Autodesk Inventor part; units mm, degrees
ref_plane "工作平面2" through (0, 56, 0) normal (0, 1, 0) x (1, 0, 0)
ref_plane "YZ Plane" through (0, 0, 0) normal (1, 0, 0) x (0, 1, 0)
ref_plane "XZ Plane" through (0, 0, 0) normal (0, 1, 0) x (-1, 0, 0)
sketch "草图1" plane through (0, 0, 0) normal (0, 1, 0) x (-1, 0, 0)
  circle A0 centre (0, 0) radius 35.5
  dimension "d0" = 71
extrude "拉伸1" add sketch "草图1" along normal blind 3
sketch "草图2" plane through (0, 3, 0) normal (0, 1, 0) x (1, 0, 0)
  circle A0 centre (0, 0) radius 15.5
  circle A1 centre (0, 0) radius 12.5
  dimension "d3" = 31
  dimension "d4" = 25
extrude "拉伸2" add sketch "草图2" along normal blind 41
sketch "草图3" plane through (0, 44, 0) normal (0, 1, 0) x (1, 0, 0)
  circle A0 centre (0, 0) radius 30
  dimension "d7" = 60
extrude "拉伸3" add sketch "草图3" along normal blind 3
sketch "草图4" plane through (0, 0, 0) normal (0, -1, 0) x (1, 0, 0)
  circle A0 centre (0, 0) radius 12.5
extrude "拉伸4" cut sketch "草图4" against normal blind 3
sketch "草图5" plane through (0, 47, 0) normal (0, 1, 0) x (1, 0, 0)
  circle A0 centre (0, 0) radius 12.5
  circle A1 centre (0, 0) radius 3.5
  dimension "d12" = 7
extrude "拉伸5" cut sketch "草图5" against normal blind 5 contours A1
sketch "草图6" plane through (0, 47, 0) normal (0, 1, 0) x (1, 0, 0)
  circle A0 centre (0, 0) radius 10
  circle A1 centre (0, 0) radius 22.5
  dimension "d15" = 20
  dimension "d16" = 45
extrude "拉伸6" add sketch "草图6" along normal blind 10
sketch "草图7" plane through (0, 47, 0) normal (0, 1, 0) x (1, 0, 0)
  circle A0 centre (0, 0) radius 3.5
  line L0 (3.5, 3.5) -> (48.5, 3.5)
  line L1 (48.5, 3.5) -> (48.5, -3.5)
  line L2 (48.5, -3.5) -> (3.5, -3.5)
  line L3 (3.5, -3.5) -> (3.5, 3.5)
  dimension "d19" = 45
  dimension "d20" = 7
extrude "拉伸7" [suppressed]
sketch "草图8" plane through (0, 47, 0) normal (0, 1, 0) x (1, 0, 0)
  circle A0 centre (44.1819, 0) radius 2.5
  point P0 (0, 0)
  dimension "d23" = 5
extrude "拉伸8" [suppressed]
pattern_circular "环形阵列1" [suppressed]
sketch "草图9" plane through (0, 47, 0) normal (0, 1, 0) x (1, 0, 0)
  line L0 (24, -2.5) -> (29, -2.5)
  line L1 (29, -2.5) -> (29, 2.5)
  line L2 (29, 2.5) -> (24, 2.5)
  line L3 (24, 2.5) -> (24, -2.5)
  line L4 (-49.7, 0) -> (49.7, 0)
  point P0 (0, 0)
  dimension "d32" = 5
  dimension "d33" = 5
  dimension "d34" = 24
extrude "拉伸9" add sketch "草图9" along normal blind 16
sketch "草图10" plane through (0, 44, 0) normal (0, -1, 0) x (1, 0, 0)
  line L0 (13.5, 10) -> (26.5, 10)
  line L1 (26.5, 10) -> (26.5, -12)
  line L2 (26.5, -12) -> (13.5, -12)
  line L3 (13.5, -12) -> (13.5, 10)
  point P0 (0, 0)
  dimension "d36" = 10
  dimension "d38" = 22
  dimension "d40" = 13
  dimension "d41" = 13.5
extrude "拉伸10" cut sketch "草图10" along normal blind 4
sketch "草图11" plane through (0, 44, 0) normal (0, -1, 0) x (1, 0, 0)
  circle A0 centre (0, 0) radius 12.5
  line L0 (24, 2.5) -> (29, 2.5)
  line L1 (29, 2.5) -> (29, -2.5)
  line L2 (29, -2.5) -> (24, -2.5)
  line L3 (24, -2.5) -> (24, 2.5)
  line L4 (27.5, -1) -> (27.5, 1)
  line L5 (27.5, 1) -> (25.5, 1)
  line L6 (25.5, 1) -> (25.5, -1)
  line L7 (25.5, -1) -> (27.5, -1)
  dimension "d44" = 1.5
extrude "拉伸11" cut sketch "草图11" against normal blind 17.5 contours L7 L6 L5 L4
sketch "草图12" plane through (29, 47, 2.5) normal (1, 0, 0) x (0, 0, -1)
  line L0 (1.5, 14.5) -> (3.5, 14.5)
  line L1 (3.5, -3) -> (3.5, 14.5)
  line L2 (1.5, 14.5) -> (3.5, 14.5)
  line L3 (3.5, 14.5) -> (3.5, 12.5)
  line L4 (3.5, 12.5) -> (1.5, 12.5)
  line L5 (1.5, 12.5) -> (1.5, 14.5)
  point P0 (2.5, -47)
  dimension "d47" = 2
extrude "拉伸12" cut sketch "草图12" against normal blind 2
sketch "草图13" plane through (0, 0, 0) normal (0, -1, 0) x (1, 0, 0)
  line L0 (24, -2.5) -> (29, -2.5)
  line L1 (9, 2.3127) -> (18, 2.3127)
  line L2 (18, 2.3127) -> (18, -2.5)
  line L3 (18, -2.5) -> (9, -2.5)
  line L4 (9, -2.5) -> (9, 2.3127)
  point P0 (0, 0)
  dimension "d52" = 9
  dimension "d53" = 9
extrude "拉伸13" cut sketch "草图13" against normal blind 3
ref_plane "工作平面2" through (0, 56, 0) normal (0, 1, 0) x (1, 0, 0)
sketch "草图14" plane through (0, 57, 0) normal (0, 1, 0) x (1, 0, 0)
  circle A0 centre (0, 0) radius 10
  circle A1 centre (0, 0) radius 22.5
  arc A2 (13.5, -7.6158) -> (13.5, 7.6158) centre (0, 0) ccw
  arc A3 (13.5, 7.6158) -> (13.5, -7.6158) centre (0, 0) ccw
  circle A4 centre (0, 0) radius 21.5
  arc A5 (14.371, -8.1071) -> (14.371, 8.1071) centre (0, 0) ccw
  arc A6 (14.371, 8.1071) -> (14.371, -8.1071) centre (0, 0) ccw
  dimension "d56" = 1
sketch "草图15" plane through (0, 56, 0) normal (0, 1, 0) x (1, 0, 0)
  circle A0 centre (0, 0) radius 10
  circle A1 centre (0, 0) radius 22.5
  arc A2 (13.5, -7.6158) -> (13.5, 7.6158) centre (0, 0) ccw
  arc A3 (13.5, 7.6158) -> (13.5, -7.6158) centre (0, 0) ccw
  circle A4 centre (0, 0) radius 21.5
  arc A5 (14.371, -8.1071) -> (14.371, 8.1071) centre (0, 0) ccw
  arc A6 (14.371, 8.1071) -> (14.371, -8.1071) centre (0, 0) ccw
  dimension "d58" = 1
extrude "拉伸14" cut sketch "草图15" against normal blind 10 contours A4
properties part number "电机帽" material "尼龙 6/6"
Model file for the job. Use its own axes, mm. A direction names the side the tool comes from. Coordinates: 2 decimals unless noted, no trailing zeros. Loops run counter-clockwise (first coordinate to the right, second up) from the corner with the lowest first, then second, coordinate; pieces in that order, holes last. Notation, with made-up numbers: (-1, -3.75) -> (42, -3.75) arc R24 cw to (42, 34.25) -> close; hole circle Ø6 at (46.25, 9). An arc over 180 degrees is marked (long way). Use one line per item in the form item = value. Start each with the question number.
(1) Probe probe 1 along Y at (x, z) = (18.5, 4); probe 2 along X at (y, z) = (53, 0); probe 3 along X at (y, z) = (45.3, 0). List the from-to ranges inside material, lowest first. Write a range as from..to.
(2) Tool access for faces 4 (the flat face through (14, 3, 0)), 5 (the flat face through (27, 61.5, 0)), 6 (the flat face through (29, 55, 0)): list every direction of +Z, -Z, +X, -X, +Y, -Y with a clear straight run to the whole face (end or side of a thin tool).
(3) Cut at C-C on z = 0. Give the number of separate pieces and of enclosed holes in the cut face, and give its area (4 significant figures).
(4) Flat gauge pins, fed straight in: pin 1 (1 mm diameter, centred on x = -21.5, z = 22.5, fed in from +Y); pin 2 (9 mm diameter, centred on x = 0, z = 0, fed in from -Y); pin 3 (21.5 mm diameter, centred on x = -4.5, z = -2.5, fed in from +Y); pin 4 (8 mm diameter, centred on y = 26.5, z = -20, fed in from -X). Where does each tip first touch, or does it go through?
(5) Cut at A-A on y = 53.5. Give the cut face in (x, z).
(6) Pull direction Z, two halves, no side cores. Call faces 1 (the flat face through (27, 55, -2.5)), 2 (the flat face through (26, 53, 1)), 3 (the flat face through (-22.4, 47, -4.6)): pulls with the +Z half, pulls with the -Z half, needs draft (parallel to the pull), parting line crosses it, or undercut.
(7) Cut at B-B on z = 29. Give the cut face in (x, y), and give its area (3 significant figures).
Values:
q1.probe_1 = 0..3, 44..46, 56..57
q1.probe_2 = -22.5..-21.5, -16.5..-10, 10..16.5, 21.5..22.5, 24..25.5, 27.5..29
q1.probe_3 = -30..-3.5, 3.5..25.5, 27.5..30
q2.face_4 = -Y
q2.face_5 = +X
q2.face_6 = +Z, -Z, +X, +Y
q3.separate_pieces = 4
q3.enclosed_holes = 2
q3.area = 710.5 mm2
q4.pin_1 = 3
q4.pin_2 = 44
q4.pin_3 = 57
q4.pin_4 = through
q5.outline = circle Ø45 at (0, 0); circle Ø33 at (0, 0); (24, -2.5) -> (29, -2.5) -> (29, 2.5) -> (24, 2.5) -> close; hole circle Ø43 at (0, 0); hole circle Ø20 at (0, 0); hole (25.5, -1) -> (27.5, -1) -> (27.5, 1) -> (25.5, 1) -> close
q6.face_1 = pulls with the -Z half
q6.face_2 = undercut
q6.face_3 = needs draft
q7.outline = (-20.48, 0) -> (20.48, 0) -> (20.48, 3) -> (-20.48, 3) -> close; (-7.68, 44) -> (7.68, 44) -> (7.68, 47) -> (-7.68, 47) -> close
q7.area = 169 mm2
